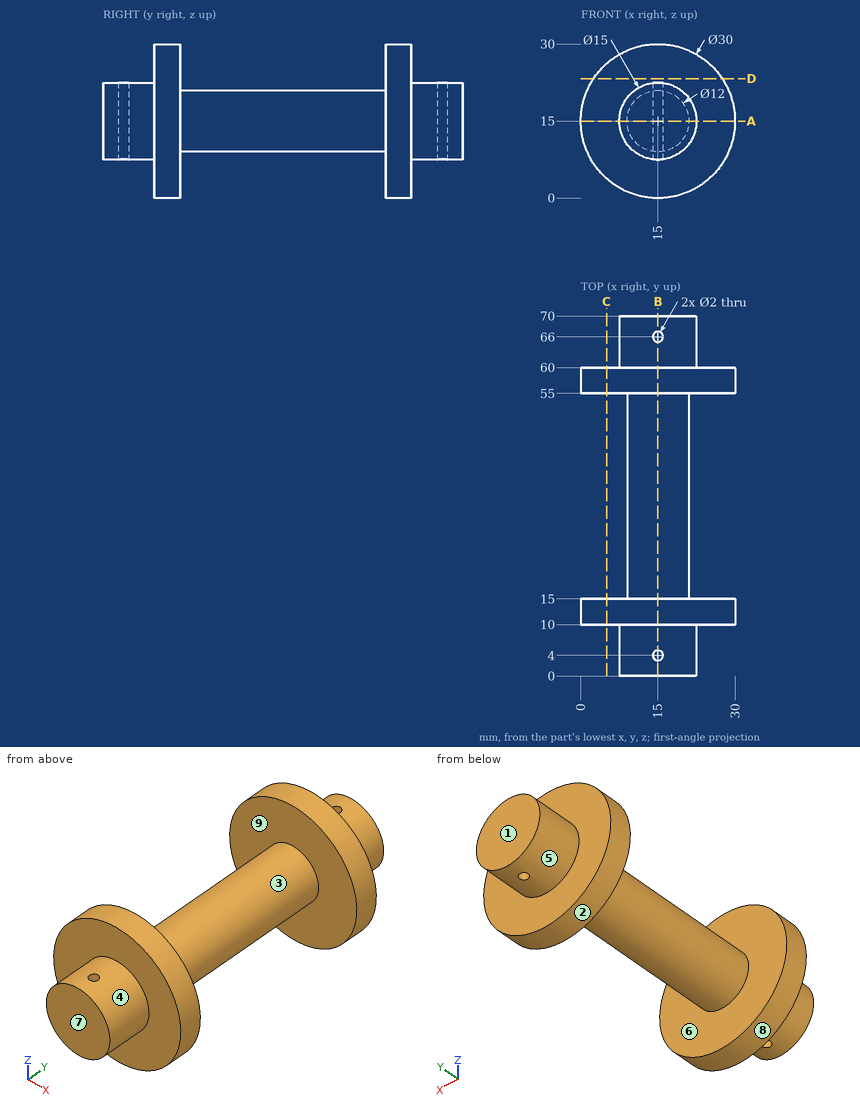
Geometry: see drawing. Coordinates: mm, zero at the bounding-box minimum. A direction names the side the tool comes from. Round coordinates to 2 decimals unless told otherwise and drop trailing zeros. Write each loop counter-clockwise with the first axis right and the second up, starting at its lowest first coordinate (ties: lowest second). Pieces come first, ordered by that corner, then holes. Notation, with made-up numbers: M 39.5,52 L 55.5,52 A25 ccw 55.5,64 Z; hole C 37.5,26.25 d4. An arc over 180 degrees is marked long. Answer in a Markdown table with one row per item. Add a question column.
(1) Reachability of the marked faces 1, 2, 3, 4 and 5 from +Z, -Z, +X, -X, +Y, -Y: full face, straight path, thin tool, end or side. Return the list, or none.
(2) Cut plane B-B, the plane x = 15. Return the cut outline in (y, z), then the cut area to 3 significant figures.
(3) Cut plane A-A, the plane z = 15. Return the cut outline in (x, y), then the cut area to 3 significant figures.
(4) Draft query along Y for the marked faces 6, 7, 8 and 9. Return one class per face: pulls with the +Y half, pulls with the -Y half, needs draft (parallel to the pull), parting line crosses it, or undercut.
(5) Cut plane D-D, the plane z = 23.25. Return the cut outline in (x, y).
(6) Contact query for flat-ended pins moving along their axis: pin 1 (12 mm diameter, centred on x = 6.5, y = 15, fed in from +Z); pin 2 (2 mm diameter, centred on y = 28.5, z = 10, fed in from +X); pin 3 (10 mm diameter, centred on x = 7, z = 25, fed in from +Y). Output: stop coordinate, or through.
(7) Ray query, L1, parallel to Y at x = 15, z = 15.75; L2, parallel to Y at x = 16.75, z = 2; L3, parallel to Z at x = 21.25, y = 63.5. Return the intervals inside material, ascending.
(8) Cut plane C-C, the plane x = 5. Return the cut outline in (y, z), then the cut area to 3 significant figures.
Established:
| question | item | result |
|---|---|---|
| 1 | face 1 | +Z, -Z, +X, -X, +Y |
| 1 | face 2 | +Y, -Y |
| 1 | face 3 | none |
| 1 | face 4 | -Y |
| 1 | face 5 | +Y |
| 2 | outline | M 0,7.5 L 3,7.5 L 3,22.5 L 0,22.5 Z; M 5,7.5 L 10,7.5 L 10,0 L 15,0 L 15,9 L 55,9 L 55,0 L 60,0 L 60,7.5 L 65,7.5 L 65,22.5 L 60,22.5 L 60,30 L 55,30 L 55,21 L 15,21 L 15,30 L 10,30 L 10,22.5 L 5,22.5 Z; M 67,7.5 L 70,7.5 L 70,22.5 L 67,22.5 Z |
| 2 | area | 1,020 mm² |
| 3 | outline | M 0,10 L 7.5,10 L 7.5,0 L 22.5,0 L 22.5,10 L 30,10 L 30,15 L 21,15 L 21,55 L 30,55 L 30,60 L 22.5,60 L 22.5,70 L 7.5,70 L 7.5,60 L 0,60 L 0,55 L 9,55 L 9,15 L 0,15 Z; hole C 15,4 d2; hole C 15,66 d2 |
| 3 | area | 1,070 mm² |
| 4 | face 6 | undercut |
| 4 | face 7 | pulls with the -Y half |
| 4 | face 8 | needs draft |
| 4 | face 9 | undercut |
| 5 | outline | M 2.47,10 L 27.53,10 L 27.53,15 L 2.47,15 Z; M 2.47,55 L 27.53,55 L 27.53,60 L 2.47,60 Z |
| 6 | pin 1 | z = 29.79 |
| 6 | pin 2 | x = 19.47 |
| 6 | pin 3 | y = 60 |
| 7 | L1 | 0 to 3, 5 to 65, 67 to 70 |
| 7 | L2 | 10 to 15, 55 to 60 |
| 7 | L3 | 10.85 to 19.15 |
| 8 | outline | M 10,3.82 L 15,3.82 L 15,26.18 L 10,26.18 Z; M 55,3.82 L 60,3.82 L 60,26.18 L 55,26.18 Z |
| 8 | area | 224 mm² |
